Model file for the job. Use its own axes, mm. Face numbers are marked on the shaded views. Coordinates: 2 decimals unless noted, no trailing zeros. Write each loop counter-clockwise with the first axis right and the second up, starting at its lowest first coordinate (ties: lowest second). Pieces come first, ordered by that corner, then holes.
Q1. Band-saw the part on D-D, the plane y = 12.5. Write the cut outline in (x, z).
Q2. Band-saw the part on A-A, the plane x = 0. Write the cut outline in (y, z), plus the area to 3 significant figures.
Q3. Band-saw the part on B-B, the plane z = 0. Write the cut outline in (x, y).
Q4. Pull direction X, two halves, no side cores. Call the marked faces 1, 2 and 3: released by +X, released by -X, zero draft, split by the parting line, or undercut.
Q5. Band-saw the part on C-C, the plane y = 45. Write the cut outline in (x, z).
Q6. Pin check, flat tips, straight feed: P1, Ø10, axis at x = 13, y = 56, coming from the +Z side; P2, Ø22, axis at x = -3.5, z = 1.5, coming from the +Y side; P3, Ø1, axis at x = 10, y = 61.5, coming from the +Z side; P4, Ø6, axis at x = -14, z = -3.5, coming from the -Y side. Stop position of each tip, or through.
Q7. Drill centre lines: probe 1 along Y at (x, z) = (-13, 5.5); probe 2 along Z at (x, y) = (3, 33.5); probe 3 along X at (y, z) = (61, -9). Where is each one in solid material? Low to high.
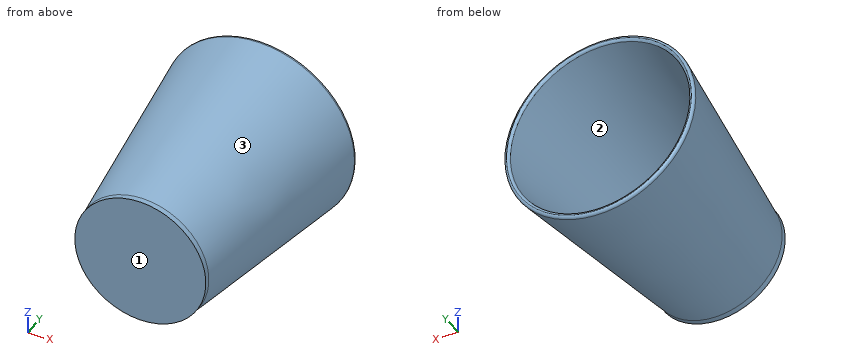
from build123d import *

# Parameters (mm, degrees)
CROQUIS1_R              = 24
SALIENTE_EXTRUIR1_DEPTH = 2
REDONDEO1_R             = 1
REDONDEO2_R             = 1


with BuildPart() as part:
    # Croquis1 → Saliente-Extruir1 (new body)
    with BuildSketch(Plane(origin=(0, 0, 0), x_dir=(1, 0, 0), z_dir=(0, 1, 0))):
        with Locations(Location((0, 0, 0), (0, 0, 270))):
            Circle(CROQUIS1_R)
    extrude(amount=SALIENTE_EXTRUIR1_DEPTH)

    # Croquis2 → Revolución1 (revolve)
    with BuildSketch(Plane.XY, mode=Mode.PRIVATE) as revoluci_n1_sk:
        Polygon((24, 2), (35, 80), (33, 80), (22, 2), align=None)
    revolve(revoluci_n1_sk.sketch.rotate(Axis((0, 2, 0), (0, 1, 0)), 270), axis=Axis((0, 2, 0), (0, 1, 0)))

    # Redondeo1
    redondeo1_edges = [part.edges().sort_by_distance(p)[0] for p in [
        (0, 80, -35),
    ]]
    fillet(redondeo1_edges, radius=REDONDEO1_R)

    # Redondeo2
    # the kernel refuses this fillet: 1 mm, written as the material it takes off along each edge
    with BuildSketch(Plane(origin=(0, 80, 0), x_dir=(0, 0, 1), z_dir=(-1, 0, 0))) as redondeo2_piece_1:
        with BuildLine():
            CenterArc((33 + REDONDEO2_R * 0.868869517606, -REDONDEO2_R), REDONDEO2_R, 90, 81.97276249)
            Line((33 - REDONDEO2_R * 0.121332278545, -REDONDEO2_R * 0.860356156953), (33, 0))
            Line((33, 0), (33 + REDONDEO2_R * 0.868869517606, 0))
        make_face()
    revolve(axis=Axis((0, 80, 0), (0, 1, 0)), mode=Mode.SUBTRACT)


solid = part.part
Answer sheet:
1. outline: circle Ø50.96 at (0, 0); hole circle Ø46.96 at (0, 0)
2. outline: (0, -24) - (2, -24) - (78.86, -34.84) arc R1 ccw to (80, -33.86) arc R1 ccw to (79.14, -32.88) - (2, -22) - (2, 22) - (79.14, 32.88) arc R1 ccw to (80, 33.86) arc R1 ccw to (78.86, 34.84) - (2, 24) - (0, 24) - close
2. area: 407 mm2
3. outline: (-34.84, 78.86) - (-24, 2) - (-24, 0) - (24, 0) - (24, 2) - (34.84, 78.86) arc R1 ccw to (33.86, 80) arc R1 ccw to (32.88, 79.14) - (22, 2) - (-22, 2) - (-32.88, 79.14) arc R1 ccw to (-33.86, 80) arc R1 ccw to start
4. face 1: zero draft
4. face 2: undercut
4. face 3: split by the parting line
5. outline: circle Ø60.13 at (0, 0); hole circle Ø56.13 at (0, 0)
6. P1: stops at z = 30.77
6. P2: stops at y = 2
6. P3: stops at z = 30.98
6. P4: stops at y = 0
7. probe 1: y = 0 to 2
7. probe 2: z = -28.28 to -26.27, 26.27 to 28.28
7. probe 3: x = -31.04 to -28.95, 28.95 to 31.04
